Autodesk Fusion 360 part; units mm, degrees
sketch "Szkic1" plane through (0, 0, 0) normal (0, 0, 1) x (1, 0, 0)
  line L0 (160, 60) -> (-160, 60)
  line L1 (-160, 60) -> (-160, -60)
  line L2 (-160, -60) -> (160, -60)
  line L3 (160, -60) -> (160, 60)
  line L4 (160, 60) -> (-160, -60) construction
  line L5 (-160, 60) -> (160, -60) construction
  dimension "d1" = 120
  dimension "d2" = 320
extrude "Wyciągnięcie proste1" add sketch "Szkic1" along normal blind 8
sketch "Szkic2" plane through (0, 0, 0) normal (0, 1, 0) x (1, 0, 0)
  line L0 (107.5, -8) -> (107.5, -20.5)
  line L1 (107.5, -20.5) -> (132.5, -20.5)
  line L2 (132.5, -20.5) -> (132.5, -8)
  circle A0 centre (120, -20.5) radius 12.5
  line L3 (107.5, -8) -> (132.5, -8)
  line L4 (-160, -8) -> (160, -8)
  circle A1 centre (120, -20.5) radius 7.5
  dimension "d5" = 15
  dimension "d6" = 25
  dimension "d7" = 40
extrude "Wyciągnięcie proste2" add sketch "Szkic2" against normal blind 20 from surface at 50 contours L0 A0 L3 L4 | L1 A0 A1 | L1 A0 A1 | L2 A0 L3 L4
sketch "Szkic4" plane through (0, 0, 0) normal (1, 0, 0) x (0, 1, 0)
  line L0 (19, 8) -> (19, 18)
  arc A0 (24, 23) -> (19, 18) centre (24, 18) ccw
  line L1 (29, 18) -> (29, 16)
  arc A1 (29, 18) -> (24, 23) centre (24, 18) ccw
  point P0 (19, 23)
  point P1 (29, 23)
  dimension "d11" = 15
  dimension "d12" = 10
  dimension "d13" = 5
  dimension "d23" = 7
  dimension "d24" = 5
ref_plane "Płaszczyzna konstrukcyjna1" through (0, 29, 0) normal (0, 1, 0) x (0, 0, 1)
sketch "Szkic6" plane through (0, 0, 8) normal (0, 0, 1) x (-1, 0, 0)
  circle A0 centre (0, -19) radius 3
  circle A1 centre (0, -19) radius 5
  line L0 (-132.5, -50) -> (-132.5, -30)
  line L1 (-132.5, -30) -> (-107.5, -30)
  line L2 (-107.5, -30) -> (-107.5, -50)
  line L3 (-107.5, -50) -> (-132.5, -50)
  line L4 (-160, 60) -> (-160, -60)
  line L5 (-160, -60) -> (160, -60)
  line L6 (160, -60) -> (160, 60)
  line L7 (160, 60) -> (-160, 60)
  point P0 (0, -19)
  dimension "d14" = 10
  dimension "d15" = 6
sweep "Przeciągnięcie2" add profiles "Szkic6" path "Szkic4" along L1 A1 A0 L0 section 1 contours A0
mirror "Odbij1" about plane through (0, 0, 0) normal (0, 1, 0) of "Wyciągnięcie proste2", "Przeciągnięcie2"
sketch "Szkic7" plane through (0, 0, 8) normal (0, 0, 1) x (-1, 0, 0)
sketch "Szkic8" plane through (0, 0, 8) normal (0, 0, 1) x (-1, 0, 0)
  circle A0 centre (135, 20) radius 5
  line L0 (160, -60) -> (160, 60)
  line L1 (-160, -60) -> (160, -60)
  line L2 (0, 0) -> (60, 0)
  circle A1 centre (135, 20) radius 9
  dimension "d33" = 10
  dimension "d34" = 25
  dimension "d38" = 80
  dimension "d39" = 18
extrude "Wyciągnięcie proste3" add sketch "Szkic8" along normal blind 10 contours A0 | A1
extrude "Wyciągnięcie proste4" add sketch "Szkic8" along normal blind 25 contours A0
For this review, take the finished solid that the model builds, in its own axes (mm). A direction names the side the tool comes from. Coordinates: 2 decimals unless noted, no trailing zeros. Write each loop counter-clockwise with the first axis right and the second up, starting at its lowest first coordinate (ties: lowest second). Pieces come first, ordered by that corner, then holes. Notation, with made-up numbers: (-26.5, 39) -> (23.5, 39) arc R19 ccw to (23.5, 70) -> close; hole circle Ø5 at (16, 6). An arc over 180 degrees is marked (long way). Write each question's results on one line, items separated by ' | '. Start each with the question number.
1) Consider section C-C (y = 10). Write out the cut boundary in (x, z), plus the area to 3 significant figures.
2) Consider section B-B (x = -135). Write out the cut boundary in (y, z), plus the area to 3 significant figures.
3) For faces 4 (the face through (0.65, 21.93, 13.07)), 5 (the face through (125.4, 50, 14.8)), 6 (the face through (-139, -16, 18)), 7 (the face through (132.5, 40, 14)), 8 (the face through (125.4, 30, 14.8)), list the 3-axis set-ups (+Z, -Z, +X, -X, +Y, -Y) from which the entire face can be reached by the end or side of a thin tool; tool diameter is ignored.
4) Wall thickness on L1, parallel to X at y = 41.5, z = 20.5; L2, parallel to Z at x = 120, y = -41; L3, parallel to X at y = -20, z = 21.5: over which ranges is each line inside the solid? List them lowest first. Write a range as [from, to].
5) The part is to be moulded in two halves that separate along Z. For faces 1 (the face through (107.5, -40, 14)), 2 (the face through (120, 40, 33)), 3 (the face through (0, 29, 16)), say which applies: +Z half, -Z half, draft (parallel to the pull), parting line (faces both ways), or undercut.
6) Consider section A-A (x = 120). Write out the cut boundary in (y, z), plus the area to 3 significant figures.
7) Consider section D-D (x = 64). Write out the cut boundary in (y, z), plus the area to 3 significant figures.
8) Insertion check: pin 1 (19.5 mm diameter, centred on x = 120, z = 20.5, fed in from +Y); pin 2 (6 mm diameter, centred on y = 40.5, z = 12.5, fed in from +X); pin 3 (12 mm diameter, centred on x = 27, y = -32.5, fed in from +Z). Each pin has a flat end and moves straight along its axis. Give the tip position at first contact, or say it passes through.
Geometry says:
1) outline: (-160, 0) -> (160, 0) -> (160, 8) -> (-160, 8) -> close | area: 2,560 mm^2
2) outline: (-60, 0) -> (60, 0) -> (60, 8) -> (-11, 8) -> (-11, 18) -> (-15, 18) -> (-15, 33) -> (-25, 33) -> (-25, 18) -> (-29, 18) -> (-29, 8) -> (-60, 8) -> close | area: 1,290 mm^2
3) face 4: none | face 5: +Z, +X, -X, +Y | face 6: +Z | face 7: +Z, +X, +Y, -Y | face 8: +Z, +X
4) L1: [107.5, 112.5], [127.5, 132.5] | L2: [0, 13], [28, 33] | L3: [-140, -130], [-2.98, 2.98]
5) face 1: draft | face 2: +Z half | face 3: undercut
6) outline: (-60, 0) -> (60, 0) -> (60, 8) -> (50, 8) -> (50, 13) -> (30, 13) -> (30, 8) -> (-30, 8) -> (-30, 13) -> (-50, 13) -> (-50, 8) -> (-60, 8) -> close; (-50, 28) -> (-30, 28) -> (-30, 33) -> (-50, 33) -> close; (30, 28) -> (50, 28) -> (50, 33) -> (30, 33) -> close | area: 1,360 mm^2
7) outline: (-60, 0) -> (60, 0) -> (60, 8) -> (-60, 8) -> close | area: 960 mm^2
8) pin 1: y = 50 | pin 2: x = 132.5 | pin 3: z = 8
